Could you check a few things on this model? Use its own coordinates, in mm. Give positions to 0.01 mm unless a question says otherwise; leave off trailing zeros. Loops run counter-clockwise (first coordinate to the right, second up) from the corner with the lowest first, then second, coordinate; pieces in that order, holes last. Notation, with made-up numbers: M -36,5 L -28,5 A14 ccw -28,20 Z; hole C 11.5,60.25 d11. An arc over 180 degrees is marked long. Use a Markdown table: item, result. Add a question column.
1) Suppose I cut it at C-C on y = 213.5. List the corners of the cut face in (x, z) for me.
2) Suppose I cut it at A-A on z = 3.45. List the corners of the cut face in (x, y) for me (1 decimal), and give its area (3 significant figures).
3) Suppose I cut it at B-B on x = -16. List the corners of the cut face in (y, z) for me, and give its area (3 significant figures).
4) If I drill on line 1 along X through (y, z) = (96, 1.4); line 2 along X through (y, z) = (177, 3.2), over which ranges is the centre line in solid material (lowest first)? Write a range as [from, to].
5) Will this pin go through, and if not, where does the flat tip stop? pin 1 Ø8 at (x, y) = (-23.5, 149) entering from +Z.
```python
from build123d import *

# Parameters (mm, degrees)
THICKEN1_START = 0.5
THICKEN1_DEPTH = 6


# Read off the part's stored shape, not the designer's step: Thicken1
with BuildPart() as part:
    # Thicken1 outline → Thicken1 (new body)
    with BuildSketch(Plane.XY.offset(THICKEN1_START)):
        with BuildLine():
            Line((-44.084142674, 245.790557606), (-7.418638396, -1.101727894))
            ThreePointArc((-7.418638396, -1.101727894), (1.101727894, -7.418638396), (7.418638396, 1.101727894))
            Line((7.418638396, 1.101727894), (-29.246865883, 247.994013395))
            ThreePointArc((-29.246865883, 247.994013395), (-37.767232173, 254.310923896), (-44.084142674, 245.790557606))
        make_face()
        with BuildLine():
            ThreePointArc((6.42948661, 0.954830842), (0.954830842, -6.42948661), (-6.42948661, -0.954830842))
            Line((-6.42948661, -0.954830842), (-43.094990888, 245.937454659))
            ThreePointArc((-43.094990888, 245.937454659), (-37.62033512, 253.32177211), (-30.236017669, 247.847116343))
            Line((-30.236017669, 247.847116343), (6.42948661, 0.954830842))
        make_face(mode=Mode.SUBTRACT)
    extrude(amount=THICKEN1_DEPTH)


solid = part.part
```
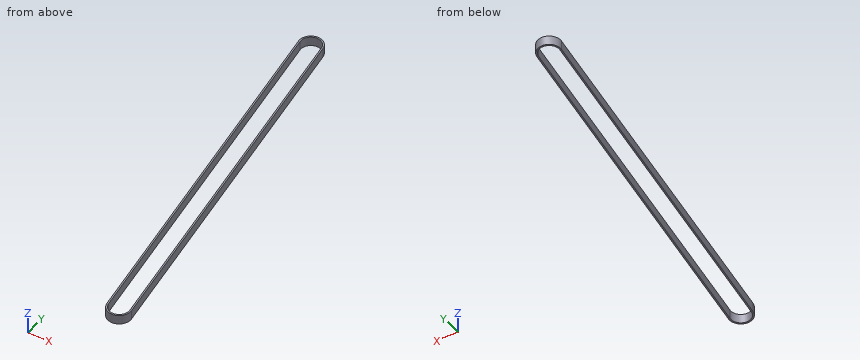
Answer block:
| question | item | result |
|---|---|---|
| 1 | outline | M -39.29,0.5 L -38.28,0.5 L -38.28,6.5 L -39.29,6.5 Z; M -25.14,0.5 L -24.12,0.5 L -24.12,6.5 L -25.14,6.5 Z |
| 2 | outline | M -44.1,245.8 L -7.4,-1.1 A7.5 ccw 7.4,1.1 L -29.2,248 A7.5 ccw Z; hole M -43.1,245.9 L -6.4,-1 A6.5 ccw 6.4,1 L -30.2,247.8 A6.5 ccw Z |
| 2 | area | 543 mm^2 |
| 3 | outline | M 56.68,0.5 L 63.49,0.5 L 63.49,6.5 L 56.68,6.5 Z; M 151.99,0.5 L 158.79,0.5 L 158.79,6.5 L 151.99,6.5 Z |
| 3 | area | 81.7 mm^2 |
| 4 | line 1 | x = [-21.84, -20.83], [-7.69, -6.67] |
| 4 | line 2 | x = [-33.87, -32.86], [-19.71, -18.7] |
| 5 | pin 1 | passes through |
